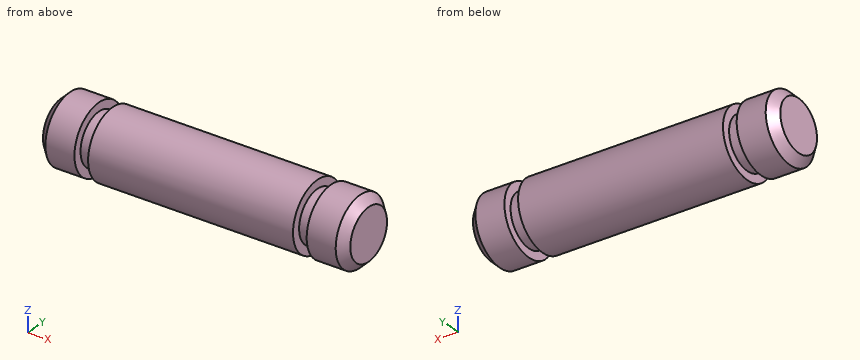
```python
from build123d import *

# Parameters (mm, degrees)
SKETCH1_R           = 2
BOSS_EXTRUDE1_DEPTH = 9
CHAMFER1_SIZE       = 0.5
CUT_EXTRUDE1_START  = -3
SKETCH2_R           = 2
SKETCH2_R_2         = 1.5
CUT_EXTRUDE1_DEPTH  = 0.8


with BuildPart() as part:
    # Sketch1 → Boss-Extrude1 (new body, symmetric)
    with BuildSketch(Plane(origin=(0, 0, 0), x_dir=(0, 0, -1), z_dir=(1, 0, 0))):
        Circle(SKETCH1_R)
    extrude(amount=BOSS_EXTRUDE1_DEPTH, both=True)

    # Chamfer1
    chamfer1_edges = [part.edges().sort_by_distance(p)[0] for p in [
        (-9, 0, 2),
        (9, 0, 2),
    ]]
    chamfer(chamfer1_edges, length=CHAMFER1_SIZE)

    # Sketch2 → Cut-Extrude1 (cut)
    with BuildSketch(Plane(origin=(9, 0, 0), x_dir=(0, 0, -1), z_dir=(1, 0, 0)).offset(CUT_EXTRUDE1_START)):
        Circle(SKETCH2_R)
        Circle(SKETCH2_R_2, mode=Mode.SUBTRACT)
    cut_extrude1 = extrude(amount=CUT_EXTRUDE1_DEPTH, mode=Mode.SUBTRACT)

    # Mirror1: Cut-Extrude1 across plane
    add(cut_extrude1.mirror(Plane(origin=(0, 0, 0), x_dir=(0, 0, 1), z_dir=(1, 0, 0))), mode=Mode.SUBTRACT)


solid = part.part
```
Check sheet for the modelled part. Datum: model origin and axes. Units: mm. Coordinates: 2 decimals unless noted, no trailing zeros. Order: outer loops, then holes, each group sorted by start corner. A loop starts at its lowest first (then second) coordinate and runs counter-clockwise, first axis right, second up. Notation, with made-up numbers: M -18,-4 L 25,-4 A21 cw 25,34 Z; hole C -9.5,82 d3. An arc over 180 degrees is marked long. One line per question, with ' | ' between items. Start each with the question number.
Item 1: Sectioned sample at A-A on y = 0. Record the cut outline in (x, z).
Item 2: Sectioned sample at C-C on y = -1.75. Count the separate pieces of the cut face and the enclosed holes in it, and give its area (3 significant figures).
Item 3: Gauge pin test, flat end, axial feed: P1, Ø1.5, axis at x = -1.5, y = 0.5, coming from the +Z side. Record the tip position at first contact, or that the pin passes through.
Item 4: Sectioned sample at D-D on x = 2.75. Record the cut outline in (y, z), and give its area (3 significant figures).
Item 5: Material ranges on line 1 (X direction, y = -1.75, z = 0.65); line 2 (X direction, y = -0.9, z = -1.3); line 3 (Y direction, x = 3.5, z = -1.15), recorded low to high.
Answer below:
1) outline: M -9,-1.5 L -8.5,-2 L -6.8,-2 L -6.8,-1.5 L -6,-1.5 L -6,-2 L 6,-2 L 6,-1.5 L 6.8,-1.5 L 6.8,-2 L 8.5,-2 L 9,-1.5 L 9,1.5 L 8.5,2 L 6.8,2 L 6.8,1.5 L 6,1.5 L 6,2 L -6,2 L -6,1.5 L -6.8,1.5 L -6.8,2 L -8.5,2 L -9,1.5 Z
2) separate pieces: 3 | enclosed holes: 0 | area: 30.5 mm^2
3) P1: stops at z = 2
4) outline: C 0,0 d4 | area: 12.6 mm^2
5) line 1: x = -8.63 to -6.8, -6 to 6, 6.8 to 8.63 | line 2: x = -8.92 to -6.8, -6 to 6, 6.8 to 8.92 | line 3: y = -1.64 to 1.64
